Geometry: final body of the model. Coordinates: model frame, mm. A direction names the side the tool comes from. Give positions to 0.01 mm unless a question says otherwise; leave off trailing zeros. Write each loop counter-clockwise with the first axis right and the second up, starting at its lowest first coordinate (ties: lowest second). Pieces come first, ordered by that corner, then holes.
Q1. Section C-C (y = 0). Return the cut outline in (x, z), plus the area to 3 significant figures.
Q2. Section A-A (z = -18). Return the cut outline in (x, y), plus the area to 3 significant figures.
Q3. Pin query (flat end, axial travel): pin 1 Ø4 at (y, z) = (2.5, -24.5) entering from -X; pin 2 Ø1 at (x, y) = (13.5, 2.5) entering from +Z; pin 3 Ø2.5 at (x, z) = (-2, -1.5) entering from +Y; pin 4 Ø2 at (y, z) = (-2, -9) entering from -X. Return the tip coordinate at first contact, or that it passes through.
Q4. Mould query, pull axis X, two halves, no side actions, for faces 1 (the flat face through (-25, -2, -6)), 2 (the cylindrical face through (-24.535, 0.112, -20.548)), 3 (the flat face through (0, 11.5, -1)). Classes: +X half, -X half, draft (parallel to the pull), parting line (faces both ways), or undercut.
Q5. Reachability of faces 4 (the cylindrical face through (-23.859, 17.797, -6.36)), 5 (the flat face through (0, -16, -5)), 6 (the flat face through (-25, -2, -26)), 7 (the cylindrical face through (-23.859, 17.797, -25.516)) from +Z, -Z, +X, -X, +Y, -Y: full face, straight path, thin tool, end or side. Return the list, or none.
Q6. Line query: line 1 (X direction, y = -10, z = -5.75); line 2 (X direction, y = -5.5, z = -2.5); line 3 (Y direction, x = 17.5, z = -26.25). Output: solid intervals per line, ascending.
Q7. Section B-B (x = 0). Return the cut outline in (y, z).
Q8. Section D-D (z = -24.5). Return the cut outline in (x, y).
from build123d import *
from build123d.topology import SkipClean

# Parameters (mm, degrees)
SKETCH_1_W          = 44
SKETCH_1_H          = 32
SKETCH_1_W_2        = 30
SKETCH_1_H_2        = 23
EXTRUDE_1_DEPTH     = 3
SKETCH_1_3_W        = 3
SKETCH_1_3_H        = 3
EXTRUDE_2_DEPTH     = 28
EXTRUDE_3_DEPTH     = 8
SKETCH_2_R          = 2.55
CUT_EXTRUDE_2_DEPTH = 61.373835392
EXTRUDE_START       = 2
SKETCH_2_3_W        = 6.2
SKETCH_2_3_H        = 38
SKETCH_2_3_R        = 2.55
EXTRUDE_4_DEPTH     = 2
SKETCH_3_W          = 50
SKETCH_3_H          = 6.2
SKETCH_3_R          = 2.55
EXTRUDE_5_DEPTH     = 2
SKETCH_3_2_R        = 2.55
CUT_EXTRUDE_3_DEPTH = 55.378304497
FILLET_2_R          = 4
FILLET_3_R          = 2
FILLET_4_R          = 4


with BuildPart() as part:
    # 草图1 → 凸台-拉伸1 (new body)
    with BuildSketch(Plane.XY):
        Rectangle(SKETCH_1_W, SKETCH_1_H)
        Rectangle(SKETCH_1_W_2, SKETCH_1_H_2, mode=Mode.SUBTRACT)
    extrude(amount=-EXTRUDE_1_DEPTH)

    # 草图1<3> → 凸台-拉伸2 (add)
    with BuildSketch(Plane.XY):
        Polygon((-22, -16), (-22, 16), (22, 16), (22, 19), (-25, 19), (-25, -16), align=None)
        with Locations((-23.5, -17.5)):
            Rectangle(SKETCH_1_3_W, SKETCH_1_3_H)
        with Locations((23.5, 17.5)):
            Rectangle(SKETCH_1_3_W, SKETCH_1_3_H)
    extrude(amount=-EXTRUDE_2_DEPTH)

    # 草图1<4> → 凸台-拉伸3 (add)
    with BuildSketch(Plane.XY):
        Polygon((25, 16), (22, 16), (22, -16), (-22, -16), (-22, -19), (25, -19), align=None)
    extrude(amount=-EXTRUDE_3_DEPTH)

    # 草图2 → 切除-拉伸2 (cut, through all)
    with BuildSketch(Plane.ZY.offset(25)):
        with Locations((-18, 0)):
            Circle(SKETCH_2_R)
    extrude(amount=-CUT_EXTRUDE_2_DEPTH, mode=Mode.SUBTRACT)

    # 草图2<3> → 凸台-拉伸4 (add)
    with BuildSketch(Plane.ZY.offset(25).offset(EXTRUDE_START)):
        with Locations((-18, 0)):
            Rectangle(SKETCH_2_3_W, SKETCH_2_3_H)
        with Locations((-18, 0)):
            Circle(SKETCH_2_3_R, mode=Mode.SUBTRACT)
    extrude(amount=-EXTRUDE_4_DEPTH)

    # 草图3 → 凸台-拉伸5 (add)
    with BuildSketch(Plane(origin=(0, 19, 0), x_dir=(1, 0, 0), z_dir=(0, 1, 0))):
        with Locations((0, 18)):
            Rectangle(SKETCH_3_W, SKETCH_3_H)
        with Locations(Location((0, 18, 0), (0, 0, 270))):
            Circle(SKETCH_3_R, mode=Mode.SUBTRACT)
    extrude(amount=EXTRUDE_5_DEPTH)

    # 草图3<2> → 切除-拉伸3 (cut, through all)
    with SkipClean():  # the faces are left unmerged after this step: merging them gives an invalid solid
        with BuildSketch(Plane(origin=(0, 19, 0), x_dir=(1, 0, 0), z_dir=(0, 1, 0))):
            with Locations(Location((0, 18, 0), (0, 0, 90))):
                Circle(SKETCH_3_2_R)
        extrude(amount=-CUT_EXTRUDE_3_DEPTH, mode=Mode.SUBTRACT)
    add(part.part.scale(1), mode=Mode.REPLACE)  # the faces are merged on a copy

    # 圆角2
    # the kernel refuses this fillet: 4 mm, written as the material it takes off along each edge
    with BuildSketch(Plane(origin=(-25, 19, -11.1), x_dir=(1, 0, 0), z_dir=(0, 0, -1))) as fillet_2_piece_1_section:
        with BuildLine():
            CenterArc((FILLET_2_R, FILLET_2_R), FILLET_2_R, 180, 90)
            Line((0, FILLET_2_R), (0, 0))
            Line((0, 0), (FILLET_2_R, 0))
        make_face()
    fillet_2_piece_1 = extrude(amount=26.9, mode=Mode.PRIVATE)
    fillet_2_piece_1 = split(fillet_2_piece_1, bisect_by=Plane(origin=(-24.094419543, 18.094419543, -14.9), z_dir=(0, 0, 1)), keep=Keep.TOP, mode=Mode.PRIVATE)
    add(fillet_2_piece_1, mode=Mode.SUBTRACT)
    with BuildSketch(Plane(origin=(-25, 19, -21.1), x_dir=(1, 0, 0), z_dir=(0, 0, -1))) as fillet_2_piece_2:
        with BuildLine():
            CenterArc((FILLET_2_R, FILLET_2_R), FILLET_2_R, 180, 90)
            Line((0, FILLET_2_R), (0, 0))
            Line((0, 0), (FILLET_2_R, 0))
        make_face()
    extrude(amount=16.9, mode=Mode.SUBTRACT)
    with BuildSketch(Plane(origin=(-25, 19, 10), x_dir=(1, 0, 0), z_dir=(0, 0, -1))) as fillet_2_piece_3:
        with BuildLine():
            CenterArc((FILLET_2_R, FILLET_2_R), FILLET_2_R, 180, 90)
            Line((0, FILLET_2_R), (0, 0))
            Line((0, 0), (FILLET_2_R, 0))
        make_face()
    extrude(amount=24.9, mode=Mode.SUBTRACT)
    with BuildSketch(Plane(origin=(-25, 19, 10), x_dir=(1, 0, 0), z_dir=(0, 0, -1))) as fillet_2_piece_4_section:
        with BuildLine():
            CenterArc((FILLET_2_R, FILLET_2_R), FILLET_2_R, 180, 90)
            Line((0, FILLET_2_R), (0, 0))
            Line((0, 0), (FILLET_2_R, 0))
        make_face()
    fillet_2_piece_4 = extrude(amount=34.9, mode=Mode.PRIVATE)
    fillet_2_piece_4 = split(fillet_2_piece_4, bisect_by=Plane(origin=(-24.094419543, 18.094419543, -21.1), z_dir=(0, 0, -1)), keep=Keep.TOP, mode=Mode.PRIVATE)
    add(fillet_2_piece_4, mode=Mode.SUBTRACT)

    # 圆角3
    # the kernel refuses this fillet: 2 mm, written as the material it adds along each edge
    with BuildSketch(Plane(origin=(-25, 15, -14.9), x_dir=(0, 0, 1), z_dir=(0, -1, 0)), Plane(origin=(-25, -19, -21.1), x_dir=(0, 0, -1), z_dir=(0, 1, 0))) as fillet_3_piece_1:
        with BuildLine():
            CenterArc((FILLET_3_R, FILLET_3_R), FILLET_3_R, 180, 90)
            Line((0, FILLET_3_R), (0, 0))
            Line((0, 0), (FILLET_3_R, 0))
        make_face()
    extrude(amount=34)
    with BuildSketch(Plane(origin=(-21, 19, -14.9), x_dir=(0, 1, 0), z_dir=(1, 0, 0))) as fillet_3_piece_2:
        with BuildLine():
            CenterArc((FILLET_3_R, FILLET_3_R), FILLET_3_R, 180, 90)
            Line((0, FILLET_3_R), (0, 0))
            Line((0, 0), (FILLET_3_R, 0))
        make_face()
    extrude(amount=46)
    with BuildSketch(Plane(origin=(-21, 15, -14.9), x_dir=(0, 1, 0), z_dir=(1, 0, 0))) as fillet_3_piece_3_section:
        with BuildLine():
            CenterArc((4 + FILLET_3_R, FILLET_3_R), FILLET_3_R, 180, 90)
            Line((4, FILLET_3_R), (4, 0))
            Line((4, 0), (4 + FILLET_3_R, 0))
        make_face()
    fillet_3_piece_3 = revolve(axis=Axis((-21, 15, -14.9), (0, 0, 1)), revolution_arc=90, mode=Mode.PRIVATE)
    fillet_3_piece_3 = split(fillet_3_piece_3, bisect_by=Plane(origin=(-25, 19.477397307, -14.620539083), z_dir=(1, 0, 0)), keep=Keep.TOP, mode=Mode.PRIVATE)
    fillet_3_piece_3 = split(fillet_3_piece_3, bisect_by=Plane(origin=(-22.217423946, 19, -14.620539083), z_dir=(0, 1, 0)), keep=Keep.TOP, mode=Mode.PRIVATE)
    add(fillet_3_piece_3)
    with BuildSketch(Plane(origin=(-21, 15, -14.9), x_dir=(0, 1, 0), z_dir=(1, 0, 0))) as fillet_3_piece_4_section:
        with BuildLine():
            CenterArc((4 + FILLET_3_R, FILLET_3_R), FILLET_3_R, 180, 90)
            Line((4, FILLET_3_R), (4, 0))
            Line((4, 0), (4 + FILLET_3_R, 0))
        make_face()
    fillet_3_piece_4 = revolve(axis=Axis((-21, 15, -14.9), (0, 0, 1)), revolution_arc=90, mode=Mode.PRIVATE)
    fillet_3_piece_4 = split(fillet_3_piece_4, bisect_by=Plane(origin=(-25, 17.874086427, -14.313906434), z_dir=(1, 0, 0)), keep=Keep.TOP, mode=Mode.PRIVATE)
    fillet_3_piece_4 = split(fillet_3_piece_4, bisect_by=Plane(origin=(-23.874086368, 19, -14.313906434), z_dir=(0, -1, 0)), keep=Keep.TOP, mode=Mode.PRIVATE)
    add(fillet_3_piece_4)
    with BuildSketch(Plane(origin=(-21, 15, -14.9), x_dir=(0, 1, 0), z_dir=(1, 0, 0))) as fillet_3_piece_5_section:
        with BuildLine():
            CenterArc((4 + FILLET_3_R, FILLET_3_R), FILLET_3_R, 180, 90)
            Line((4, FILLET_3_R), (4, 0))
            Line((4, 0), (4 + FILLET_3_R, 0))
        make_face()
    fillet_3_piece_5 = revolve(axis=Axis((-21, 15, -14.9), (0, 0, 1)), revolution_arc=90, mode=Mode.PRIVATE)
    fillet_3_piece_5 = split(fillet_3_piece_5, bisect_by=Plane(origin=(-25, 16.217423741, -14.620538996), z_dir=(-1, 0, 0)), keep=Keep.TOP, mode=Mode.PRIVATE)
    fillet_3_piece_5 = split(fillet_3_piece_5, bisect_by=Plane(origin=(-25.477396893, 19, -14.620538996), z_dir=(0, -1, 0)), keep=Keep.TOP, mode=Mode.PRIVATE)
    add(fillet_3_piece_5)
    with BuildSketch(Plane(origin=(25, 19, -21.1), x_dir=(0, 0, -1), z_dir=(-1, 0, 0))) as fillet_3_piece_6:
        with BuildLine():
            CenterArc((FILLET_3_R, -FILLET_3_R), FILLET_3_R, 90, 90)
            Line((0, -FILLET_3_R), (0, 0))
            Line((0, 0), (FILLET_3_R, 0))
        make_face()
    extrude(amount=46)
    with BuildSketch(Plane(origin=(-21, 15, -21.1), x_dir=(-1, 0, 0), z_dir=(0, -1, 0))) as fillet_3_piece_7_section:
        with BuildLine():
            CenterArc((4 + FILLET_3_R, FILLET_3_R), FILLET_3_R, 180, 90)
            Line((4 + FILLET_3_R, 0), (4, 0))
            Line((4, 0), (4, FILLET_3_R))
        make_face()
    fillet_3_piece_7 = revolve(axis=Axis((-21, 15, -21.1), (0, 0, -1)), revolution_arc=90, mode=Mode.PRIVATE)
    fillet_3_piece_7 = split(fillet_3_piece_7, bisect_by=Plane(origin=(-25, 17.874086364, -21.686093558), z_dir=(1, 0, 0)), keep=Keep.TOP, mode=Mode.PRIVATE)
    fillet_3_piece_7 = split(fillet_3_piece_7, bisect_by=Plane(origin=(-23.874086351, 19, -21.686093558), z_dir=(0, -1, 0)), keep=Keep.TOP, mode=Mode.PRIVATE)
    add(fillet_3_piece_7)
    with BuildSketch(Plane(origin=(-21, 15, -21.1), x_dir=(-1, 0, 0), z_dir=(0, -1, 0))) as fillet_3_piece_8_section:
        with BuildLine():
            CenterArc((4 + FILLET_3_R, FILLET_3_R), FILLET_3_R, 180, 90)
            Line((4 + FILLET_3_R, 0), (4, 0))
            Line((4, 0), (4, FILLET_3_R))
        make_face()
    fillet_3_piece_8 = revolve(axis=Axis((-21, 15, -21.1), (0, 0, -1)), revolution_arc=90, mode=Mode.PRIVATE)
    fillet_3_piece_8 = split(fillet_3_piece_8, bisect_by=Plane(origin=(-25, 16.217424103, -21.379460891), z_dir=(-1, 0, 0)), keep=Keep.TOP, mode=Mode.PRIVATE)
    fillet_3_piece_8 = split(fillet_3_piece_8, bisect_by=Plane(origin=(-25.477397304, 19, -21.379460891), z_dir=(0, -1, 0)), keep=Keep.TOP, mode=Mode.PRIVATE)
    add(fillet_3_piece_8)
    with BuildSketch(Plane(origin=(-21, 15, -21.1), x_dir=(-1, 0, 0), z_dir=(0, -1, 0))) as fillet_3_piece_9_section:
        with BuildLine():
            CenterArc((4 + FILLET_3_R, FILLET_3_R), FILLET_3_R, 180, 90)
            Line((4 + FILLET_3_R, 0), (4, 0))
            Line((4, 0), (4, FILLET_3_R))
        make_face()
    fillet_3_piece_9 = revolve(axis=Axis((-21, 15, -21.1), (0, 0, -1)), revolution_arc=90, mode=Mode.PRIVATE)
    fillet_3_piece_9 = split(fillet_3_piece_9, bisect_by=Plane(origin=(-25, 19.477396901, -21.379461023), z_dir=(1, 0, 0)), keep=Keep.TOP, mode=Mode.PRIVATE)
    fillet_3_piece_9 = split(fillet_3_piece_9, bisect_by=Plane(origin=(-22.217423514, 19, -21.379461023), z_dir=(0, 1, 0)), keep=Keep.TOP, mode=Mode.PRIVATE)
    add(fillet_3_piece_9)

    # 圆角4
    # the kernel refuses this fillet: 4 mm, written as the material it takes off along each edge
    with BuildSketch(Plane(origin=(-25, 21, -29.760254038), x_dir=(1, 0, 0), z_dir=(0, 0, 1))) as fillet_4_piece_1:
        with BuildLine():
            CenterArc((3.464101615, -4), FILLET_4_R, 90, 60)
            Line((0, -2), (-0.069282032, -1.96))
            ThreePointArc((-0.069282032, -1.96), (-0.08, -1), (-0.08, 0))
            Line((-0.08, 0), (0, 0.08))
            Line((0, 0.08), (3.464101615, 0.08))
            Line((3.464101615, 0.08), (3.464101615, 0))
        make_face()
    extrude(amount=23.520508076, mode=Mode.SUBTRACT)
    with BuildSketch(Plane(origin=(-27, 19, -29.760254038), x_dir=(0, -1, 0), z_dir=(0, 0, 1))) as fillet_4_piece_2:
        with BuildLine():
            CenterArc((3.464101615, 4), FILLET_4_R, 210, 60)
            Line((0, 2), (-0.069282032, 1.96))
            ThreePointArc((-0.069282032, 1.96), (-0.08, 1), (-0.08, 0))
            Line((-0.08, 0), (0, -0.08))
            Line((0, -0.08), (3.464101615, -0.08))
            Line((3.464101615, -0.08), (3.464101615, 0))
        make_face()
    extrude(amount=23.520508076, mode=Mode.SUBTRACT)


solid = part.part
Computed:
1. outline: (-27, -21.1) arc R2 cw to (-25, -23.1) - (-25, -28) - (-22, -28) - (-22, -20.55) - (-27, -20.55) - close; (-27, -15.45) - (-22, -15.45) - (-22, -3) - (-15, -3) - (-15, 0) - (-25, 0) - (-25, -12.9) arc R2 cw to (-27, -14.9) - close; (15, -3) - (22, -3) - (22, -8) - (25, -8) - (25, 0) - (15, 0) - close
1. area: 139 mm2
2. outline: (-27, -19) - (-22, -19) - (-22, -2.55) - (-27, -2.55) - close; (-27, 2.55) - (-22, 2.55) - (-22, 16) - (-2.55, 16) - (-2.55, 21) - (-21.54, 21) arc R4 ccw to (-25, 19) arc R4 ccw to (-27, 15.54) - close; (2.55, 16) - (25, 16) - (25, 21) - (2.55, 21) - close
2. area: 376 mm2
3. pin 1: stops at x = -25.09
3. pin 2: passes through
3. pin 3: stops at y = 19
3. pin 4: stops at x = -25
4. face 1: -X half
4. face 2: draft
4. face 3: undercut
5. face 4: +Z, -X, +Y
5. face 5: -Z
5. face 6: -Z, -X, +Y, -Y
5. face 7: -Z, -X, +Y
6. line 1: x = -25 to -22, 22 to 25
6. line 2: x = -25 to -15, 15 to 25
6. line 3: y = 16 to 19
7. outline: (-19, -8) - (-16, -8) - (-16, -3) - (-11.5, -3) - (-11.5, 0) - (-19, 0) - close; (11.5, -3) - (16, -3) - (16, -15.45) - (21, -15.45) - (21, -14.9) arc R2 cw to (19, -12.9) - (19, 0) - (11.5, 0) - close; (16, -28) - (19, -28) - (19, -23.1) arc R2 cw to (21, -21.1) - (21, -20.55) - (16, -20.55) - close
8. outline: (-25, -19) - (-22, -19) - (-22, 16) - (25, 16) - (25, 19) - (-21, 19) arc R4 ccw to (-25, 15) - close
